Can you work these out from the model? Positions are in its coordinate system, mm. Face numbers are marked on the shaded views. Coordinates: 2 decimals unless noted, no trailing zeros. Loops run counter-clockwise (first coordinate to the right, second up) from the corner with the lowest first, then second, coordinate; pieces in that order, holes last.
```python
from build123d import *

# Parameters (mm, degrees)
SKETCH1_R           = 14.5
SKETCH1_R_2         = 5
BOSS_EXTRUDE1_DEPTH = 6.35


with BuildPart() as part:
    # Sketch1 → Boss-Extrude1 (new body)
    with BuildSketch(Plane.XY):
        with BuildLine():
            Line((-14, -55), (14, -55))
            Line((14, -55), (14, -12.093386622))
            ThreePointArc((14, -12.093386622), (0, 18.5), (-14, -12.093386622))
            Line((-14, -12.093386622), (-14, -55))
        make_face()
        Circle(SKETCH1_R, mode=Mode.SUBTRACT)
        with Locations((0, -23)):
            Circle(SKETCH1_R_2, mode=Mode.SUBTRACT)
    extrude(amount=BOSS_EXTRUDE1_DEPTH)


solid = part.part
```
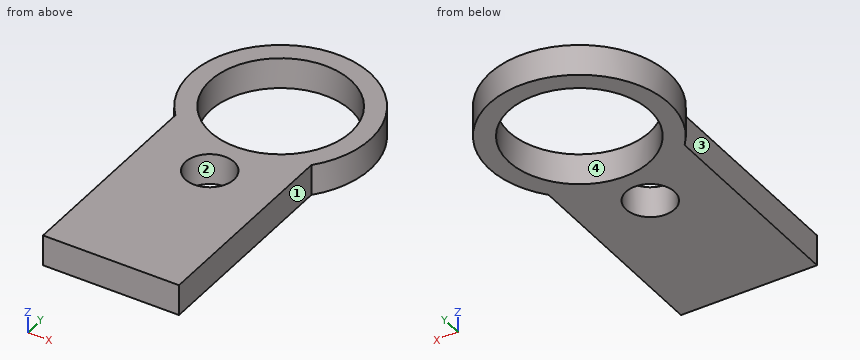
(1) If I drill on probe 1 along Y at (x, z) = (0, 4.5); probe 2 along Y at (x, z) = (-1.5, 1.5); probe 3 along Y at (x, z) = (-8.5, 3.75), over which ranges is the centre line in solid material (lowest first)?
Check values:
probe 1: y = -55 to -28, -18 to -14.5, 14.5 to 18.5
probe 2: y = -55 to -27.77, -18.23 to -14.42, 14.42 to 18.44
probe 3: y = -55 to -11.75, 11.75 to 16.43
(2) I want a section at C-C on z = 1.75. Write out the boundary of the cut face in (x, y).
Check values:
outline: (-14, -55) - (14, -55) - (14, -12.09) arc R18.5 ccw (long way) to (-14, -12.09) - close; hole circle Ø29 at (0, 0); hole circle Ø10 at (0, -23)
(3) I want a section at D-D on y = 0. Write out the boundary of the cut face in (x, z).
Check values:
outline: (-18.5, 0) - (-14.5, 0) - (-14.5, 6.35) - (-18.5, 6.35) - close; (14.5, 0) - (18.5, 0) - (18.5, 6.35) - (14.5, 6.35) - close
(4) I want a section at B-B on y = -23. Write out the boundary of the cut face in (x, z), then the cut area to 3 significant figures.
Check values:
outline: (-14, 0) - (-5, 0) - (-5, 6.35) - (-14, 6.35) - close; (5, 0) - (14, 0) - (14, 6.35) - (5, 6.35) - close
area: 114 mm2
(5) I'm going to push flat-ended pins straight in: pin 1 (1.5 mm diameter, centred on y = -36.5, z = 1, fed in from +X); pin 2 (1 mm diameter, centred on y = 1, z = 2, fed in from -X); pin 3 (17.5 mm diameter, centred on x = 0, y = 0, fed in from -Z). Where does each tip first touch, or does it pass through?
Check values:
pin 1: stops at x = 14
pin 2: stops at x = -18.49
pin 3: passes through
(6) I want a section at A-A on x = 0. Write out the boundary of the cut face in (y, z).
Check values:
outline: (-55, 0) - (-28, 0) - (-28, 6.35) - (-55, 6.35) - close; (-18, 0) - (-14.5, 0) - (-14.5, 6.35) - (-18, 6.35) - close; (14.5, 0) - (18.5, 0) - (18.5, 6.35) - (14.5, 6.35) - close
(7) If we mould it in two halves opening along X, with no side actions, what happens to the marked faces 1, 2, 3 and 4? For each: released by +X, released by -X, zero draft, split by the parting line, or undercut.
Check values:
face 1: released by +X
face 2: undercut
face 3: released by -X
face 4: undercut
